Source: CAD feature listing. Evaluate the final solid. Frame: model axes, mm. A direction names the side the tool comes from. Coordinates: 2 decimals unless noted, no trailing zeros. Loops run counter-clockwise (first coordinate to the right, second up) from the corner with the lowest first, then second, coordinate; pieces in that order, holes last. Notation, with made-up numbers: (88, 82) - (115, 82) arc R30 ccw to (115, 106) - close; hole circle Ø8 at (3.5, 82.25). An arc over 180 degrees is marked (long way). Write item = value, one per line. Start each with the question number.
from build123d import *

# Parameters (mm, degrees)
SKETCH1_R           = 1
SKETCH1_W           = 2.5
SKETCH1_H           = 20
SKETCH1_W_2         = 2.4
SKETCH1_H_2         = 16
BOSS_EXTRUDE1_DEPTH = 2.2


with BuildPart() as part:
    # Sketch1 → Boss-Extrude1 (new body)
    with BuildSketch(Plane(origin=(0, 0, 0), x_dir=(1, 0, 0), z_dir=(0, 1, 0))):
        Polygon((-117.859054558, 127.025957199), (-107.059054558, 127.025957199), (-107.059054558, 118.025957199), (-105.559054558, 118.025957199), (-105.559054558, 108.025957199), (-107.059054558, 108.025957199), (-107.059054558, 99.025957199), (-121.359054558, 99.025957199), (-121.359054558, 100.025957199), (-125.359054558, 100.025957199), (-125.359054558, 99.025957199), (-141.159054558, 99.025957199), (-141.159054558, 109.025957199), (-140.159054558, 109.025957199), (-140.159054558, 117.025957199), (-141.159054558, 117.025957199), (-141.159054558, 127.025957199), (-128.859054558, 127.025957199), (-128.859054558, 125.025957199), (-117.859054558, 125.025957199), align=None)
        with Locations(Location((-123.359054558, 111.525957199, 0), (0, 0, 270))):
            Circle(SKETCH1_R, mode=Mode.SUBTRACT)
        with Locations((-110.109054558, 114.025957199)):
            Rectangle(SKETCH1_W, SKETCH1_H, mode=Mode.SUBTRACT)
        with Locations((-136.609054558, 114.025957199)):
            Rectangle(SKETCH1_W, SKETCH1_H, mode=Mode.SUBTRACT)
        with Locations((-129.059054558, 113.025957199)):
            Rectangle(SKETCH1_W_2, SKETCH1_H_2, mode=Mode.SUBTRACT)
        with Locations((-117.659054558, 113.025957199)):
            Rectangle(SKETCH1_W_2, SKETCH1_H_2, mode=Mode.SUBTRACT)
    extrude(amount=BOSS_EXTRUDE1_DEPTH)


solid = part.part
Item 1: Cut plane C-C (x = -119.5). Return the cut outline in (y, z), then the cut area to 3 significant figures.
Item 2: First-contact query: pin 1 (0.7 mm diameter, centred on y = 1.5, z = -115, fed in from -X); pin 2 (1.1 mm diameter, centred on y = 0.5, z = -99.5, fed in from +X). Flat tips, straight axial feed; report the tip coordinate or a pass-through.
Item 3: Cut plane B-B (z = -108.5). Return the cut outline in (x, y), then the cut area to 3 significant figures.
Item 4: Reachability of faces 1 (the flat face through (-141, 1, -117.026)), 2 (the flat face through (-129, 1, -121.026)), 3 (the flat face through (-106, 1, -118.026)) from +Z, -Z, +X, -X, +Y, -Y: full face, straight path, thin tool, end or side. Return the list, or none.
Item 5: Cut plane D-D (y = 1.15). State how many separate pieces and enclosed holes the cut face has, then the cut area to 3 significant figures.
Item 6: Material intervals for L1, parallel to X at y = 1.1, z = -105.5; L2, parallel to X at y = 0.85, z = -113.25; L3, parallel to Z at x = -117, y = 1.75, sorted ascending. Write a range as [from, to].
Item 7: Draft query along Z for faces 4 (the flat face through (-130.259, 1, -113)), 5 (the flat face through (-107.059, 1, -123)), 6 (the flat face through (-106, 1, -108.026)). Return one class per face: released by +Z, released by -Z, zero draft, split by the parting line, or undercut.
Item 8: Cut plane A-A (x = -136). Return the cut outline in (y, z), then the cut area to 3 significant figures.
Responses:
q1.outline = (0, -125.03) - (2.2, -125.03) - (2.2, -99.03) - (0, -99.03) - close
q1.area = 57.2 mm2
q2.pin_1 = -140.16
q2.pin_2 = -107.06
q3.outline = (-141.16, 0) - (-137.86, 0) - (-137.86, 2.2) - (-141.16, 2.2) - close; (-135.36, 0) - (-130.26, 0) - (-130.26, 2.2) - (-135.36, 2.2) - close; (-127.86, 0) - (-118.86, 0) - (-118.86, 2.2) - (-127.86, 2.2) - close; (-116.46, 0) - (-111.36, 0) - (-111.36, 2.2) - (-116.46, 2.2) - close; (-108.86, 0) - (-105.56, 0) - (-105.56, 2.2) - (-108.86, 2.2) - close
q3.area = 56.8 mm2
q4.face_1 = -X, +Y, -Y
q4.face_2 = +Y, -Y
q4.face_3 = -Z, +X, +Y, -Y
q5.separate_pieces = 1
q5.enclosed_holes = 5
q5.area = 756 mm2
q6.L1 = [-141.16, -137.86], [-135.36, -130.26], [-127.86, -118.86], [-116.46, -111.36], [-108.86, -107.06]
q6.L2 = [-140.16, -137.86], [-135.36, -130.26], [-127.86, -118.86], [-116.46, -111.36], [-108.86, -105.56]
q6.L3 = [-127.03, -121.03], [-105.03, -99.03]
q7.face_4 = undercut
q7.face_5 = zero draft
q7.face_6 = released by +Z
q8.outline = (0, -127.03) - (2.2, -127.03) - (2.2, -124.03) - (0, -124.03) - close; (0, -104.03) - (2.2, -104.03) - (2.2, -99.03) - (0, -99.03) - close
q8.area = 17.6 mm2
